Work out the finished part from the listing and answer in its coordinate system (mm). Round coordinates to 2 decimals unless told otherwise and drop trailing zeros. Order: outer loops, then holes, each group sorted by start corner. A loop starts at its lowest first (then second) coordinate and runs counter-clockwise, first axis right, second up. Notation, with made-up numbers: (-21, -15.5) - (-11, -15.5) arc R6 cw to (-11, -4.5) - close; hole circle Ø2 at (69.25, 14.5). An arc over 180 degrees is marked (long way). Use CSV: the item, a comma, the result in double quotes.
from build123d import *

# Parameters (mm, degrees)
CROQUIS2_W                        = 2.5
CROQUIS2_H                        = 108
CROQUIS3_W                        = 7.5
CROQUIS3_H                        = 2.5
DI_METRO_DE_TALADRO_5_0_5_1_D     = 5
DI_METRO_DE_TALADRO_5_0_5_1_DEPTH = 15
CHAFL_N1_SIZE                     = 0.747946905
CHAFL_N1_SIZE2                    = 1.053583954
CROQUIS5_R                        = 3.54
CORTAR_EXTRUIR1_DEPTH             = 61.731439717


# Read off the part's stored shape, not the designer's step: Sólido importado2
with BuildPart() as part:
    # Croquis1 → Revolución1 (revolve)
    with BuildSketch(Plane.XZ):
        Polygon((4.334336082, 118), (0, 118), (0, 0), (7.5, 0), (7.5, 113.540736), align=None)
    revolve(axis=Axis((0, 0, 118), (0, 0, -1)))

    # Croquis2 → Cortar-Revolución1 (revolve, cut)
    with BuildSketch(Plane.XZ, mode=Mode.PRIVATE) as cortar_revoluci_n1_sk:
        with Locations((1.25, 59)):
            Rectangle(CROQUIS2_W, CROQUIS2_H)
    revolve(cortar_revoluci_n1_sk.sketch.rotate(Axis((0, 0, 113), (0, 0, -1)), 180), axis=Axis((0, 0, 113), (0, 0, -1)), mode=Mode.SUBTRACT)

    # Croquis3 → Cortar-Revolución2 (revolve, cut)
    with BuildSketch(Plane.XY.offset(18), mode=Mode.PRIVATE) as cortar_revoluci_n2_sk:
        with Locations((3.75, -1.25)):
            Rectangle(CROQUIS3_W, CROQUIS3_H)
    revolve(cortar_revoluci_n2_sk.sketch.rotate(Axis((7.5, 0, 18), (-1, 0, 0)), 90), axis=Axis((7.5, 0, 18), (-1, 0, 0)), mode=Mode.SUBTRACT)

    # Diámetro de taladro Ø5.0 (5)1
    with Locations(Plane(origin=(-7.5, 0, 18), x_dir=(0, 0, -1), z_dir=(-1, 0, 0))):
        with Locations((0, 0)):
            Hole(DI_METRO_DE_TALADRO_5_0_5_1_D / 2, depth=DI_METRO_DE_TALADRO_5_0_5_1_DEPTH)

    # Chaflán1
    chafl_n1_edges = [part.edges().sort_by_distance(p)[0] for p in [
        (2.5, 0, 113),
    ]]
    chafl_n1_side = [part.faces().sort_by_distance(p)[0] for p in [
        (0, 0, 113),
    ]]
    chamfer(chafl_n1_edges, length=CHAFL_N1_SIZE, length2=CHAFL_N1_SIZE2, reference=chafl_n1_side[0])

    # Croquis5 → Cortar-Extruir1 (cut)
    with BuildSketch(Plane.XY.offset(118)):
        Circle(CROQUIS5_R)
    extrude(amount=-CORTAR_EXTRUIR1_DEPTH, mode=Mode.SUBTRACT)


solid = part.part
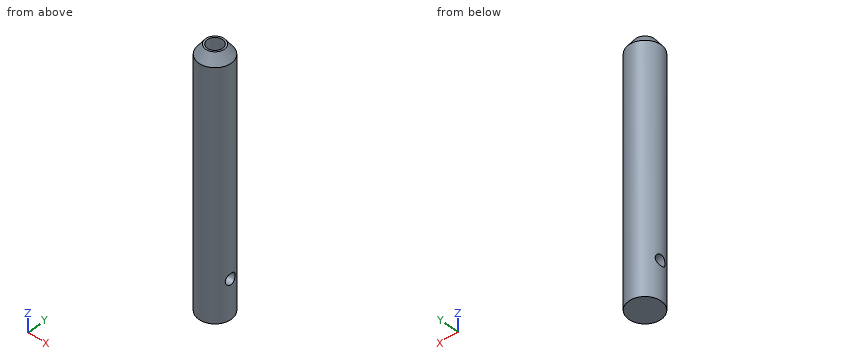
(1) Find section B-B (z = 65.5). Determine the outline of the cut face in (x, y), and give its area (3 significant figures).
Findings below:
outline,"circle Ø15 at (0, 0); hole circle Ø7.08 at (0, 0)"
area,"137 mm²"
(2) Find section A-A (y = 0). Determine the outline of the cut face in (x, z).
Findings below:
outline,"(-7.5, 0) - (7.5, 0) - (7.5, 15.5) - (2.5, 15.5) - (2.5, 5) - (-2.5, 5) - (-2.5, 15.5) - (-7.5, 15.5) - close; (-7.5, 20.5) - (-2.5, 20.5) - (-2.5, 56.27) - (-3.54, 56.27) - (-3.54, 118) - (-4.33, 118) - (-7.5, 113.54) - close; (2.5, 20.5) - (7.5, 20.5) - (7.5, 113.54) - (4.33, 118) - (3.54, 118) - (3.54, 56.27) - (2.5, 56.27) - close"
(3) Each of these flat-tipped pins is pushed along its axis until it touches: pin 1 (8 mm diameter, centred on x = -4.5, z = 46.5, fed in from -Y); pin 2 (1.5 mm diameter, centred on y = 5, z = 90, fed in from -X); pin 3 (2.5 mm diameter, centred on x = -1, y = 0, fed in from +Z). Where does it stop, or does it pass through?
Findings below:
pin 1,"stops at y = -7.48"
pin 2,"stops at x = -6.18"
pin 3,"stops at z = 5"
(4) Find section C-C (z = 39). Determine the outline of the cut face in (x, y).
Findings below:
outline,"circle Ø15 at (0, 0); hole circle Ø5 at (0, 0)"
(5) Find the intervals of material crossed by L1, parallel to X at y = 0, z = 34; L2, parallel to Z at x = 3.5, y = 0, in increasing order. Write a range as from..to.
Findings below:
L1,"x = -7.5..-2.5, 2.5..7.5"
L2,"z = 0..15.5, 20.5..56.27"
